```python
from build123d import *

# Parameters (mm, degrees)
F0_R     = 30
F0_R_2   = 25
F1_DEPTH = 25
F2_R     = 25
F2_R_2   = 10
F3_DEPTH = 10
F4_DEPTH = 20


with BuildPart() as f1:
    # F0 (on Top) → F1 (new body)
    with BuildSketch(Plane.XY):
        Circle(F0_R)
        Circle(F0_R_2, mode=Mode.SUBTRACT)
    extrude(amount=F1_DEPTH)

    # F2 (on Top) → F3 (join)
    with BuildSketch(Plane.XY):
        Circle(F2_R)
        Circle(F2_R_2, mode=Mode.SUBTRACT)
    extrude(amount=F3_DEPTH)

    # F2 (on Top) → F4 (join)
    with BuildSketch(Plane.XY):
        Circle(F2_R_2)
    extrude(amount=F4_DEPTH)


solid = f1.part
```
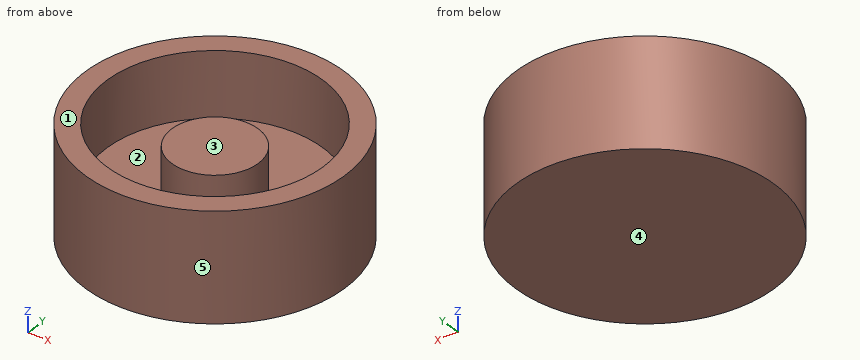
CAD build for the part. Positions are in the model's coordinates, mm. Face numbers are marked on the shaded views. A direction names the side the tool comes from. Round coordinates to 2 decimals unless told otherwise and drop trailing zeros. Order: outer loops, then holes, each group sorted by start corner. A loop starts at its lowest first (then second) coordinate and runs counter-clockwise, first axis right, second up.
Q1. Two-plate mould, pull along Y, no slides. Class the marked faces 3, 4 and 5: pulls with the +Y half, pulls with the -Y half, needs draft (parallel to the pull), parting line crosses it, or undercut.
Q2. Drop flat-ended pins along their axis: pin 1 (1.5 mm diameter, centred on x = 3, y = -8.5, fed in from +Z); pin 2 (1 mm diameter, centred on x = 4.5, y = -11, fed in from +Z); pin 3 (5 mm diameter, centred on x = -2.5, z = 12.5, fed in from +Y); pin 4 (4 mm diameter, centred on x = -18, y = -19, fed in from -Z). Give the stop position or say it passes through.
Q3. Slice it at A-A (z = 17.5). Write the cut outline in (x, y).
Q4. Slice it at B-B (y = 0). Write the cut outline in (x, z).
Q5. Slice it at D-D (z = 3.25). Write the cut outline in (x, y), and give its area (3 significant figures).
Q6. Which spindle directions (+Z, -Z, +X, -X, +Y, -Y) get a long thin tool onto all of the face, cutting with end or side? Do the marked faces 1 and 2. Say none if no direction does.
Q7. Wall check: L1, parallel to Y at x = 0, z = 18.75; L2, parallel to Y at x = -1, z = 10.5; L3, parallel to Y at x = 0, z = 21. Give the ranges that are in metal, low to high.
Results below:
1. face 3: undercut
1. face 4: needs draft
1. face 5: parting line crosses it
2. pin 1: stops at z = 20
2. pin 2: stops at z = 10
2. pin 3: stops at y = 30
2. pin 4: stops at z = 0
3. outline: circle Ø60 at (0, 0); circle Ø20 at (0, 0); hole circle Ø50 at (0, 0)
4. outline: (-30, 0) - (30, 0) - (30, 25) - (25, 25) - (25, 10) - (10, 10) - (10, 20) - (-10, 20) - (-10, 10) - (-25, 10) - (-25, 25) - (-30, 25) - close
5. outline: circle Ø60 at (0, 0)
5. area: 2,830 mm2
6. face 1: +Z, +X, -X, +Y, -Y
6. face 2: +Z
7. L1: y = -30 to -25, -10 to 10, 25 to 30
7. L2: y = -29.98 to -24.98, -9.95 to 9.95, 24.98 to 29.98
7. L3: y = -30 to -25, 25 to 30
